Source: CAD feature listing. Evaluate the final solid. Frame: model axes, mm. A direction names the side the tool comes from. Coordinates: 2 decimals unless noted, no trailing zeros. Write each loop counter-clockwise with the first axis right and the second up, starting at its lowest first coordinate (ties: lowest second). Pieces come first, ordered by that corner, then holes. Notation, with made-up numbers: M -10.75,2.5 L 16.25,2.5 A10 ccw 16.25,12.5 Z; hole C -13,74 d9. An arc over 180 degrees is marked long. One line per item, written item: value. Start each with the question number.
Item 1: Cut plane A-A, the plane x = 0. Output: boundary loops of the cut face in (y, z), then the cut area to 3 significant figures.
Item 2: Set-up query: faces 1 (the cylindrical face through (-1.73, -7.81, 107.76)), 2 (the cylindrical face through (-1.64, -7.37, 54.3)). Return all of +Z, -Z, +X, -X, +Y, -Y with unobstructed straight access to the full face (end or side cutting, diameter ignored); none if empty.
Item 3: Pin query (flat end, axial travel): P1, Ø4, axis at x = -4, z = 14.5, coming from the -Y side; P2, Ø4, axis at y = -6.5, z = 60.5, coming from the +X side; P3, Ø2, axis at y = 6.5, z = 64, coming from the +X side. Return the tip coordinate at first contact, or that it passes through.
Item 4: Cut plane C-C, the plane z = 8. Output: boundary loops of the cut face in (x, y).
Item 5: Ray query, L1, parallel to Y at x = 0, z = 107.1; L2, parallel to Y at x = 0.5, z = 53; L3, parallel to X at y = -5.75, z = 26. Return the intervals inside material, ascending. Write a range as from..to.
Item 6: Mould query, pull axis X, two halves, no side actions, for faces 3 (the cylindrical face through (-1.73, -7.81, 2.31)), 4 (the flat face through (-2, 8, 110)), 5 (the cylindrical face through (5.161, 8.095, 54.23)). Classes: released by +X, released by -X, zero draft, split by the parting line, or undercut.
```python
from build123d import *

# Parameters (mm, degrees)
F0_R         = 9.6
F0_R_2       = 8
F1_DEPTH     = 110
F0_R_3       = 7.55
F2_DEPTH     = 106
F3_DEPTH     = 4
F4_S5_R      = 8
F4_T6_DEPTH  = 14
F4_S11_R     = 8
F4_T12_DEPTH = 14


# Not quite as in the source:
# - a fillet or chamfer that OpenCascade refuses, or shapes differently, is made with other operations: its cross-section is extruded or revolved along the edge and cut away or added


with BuildPart() as f1:
    # F0 (on Top) → F1 (new body)
    with BuildSketch(Plane.XY):
        Circle(F0_R)
        Circle(F0_R_2, mode=Mode.SUBTRACT)
    extrude(amount=F1_DEPTH)

    # F0 (on Top) → F2 (join)
    with BuildSketch(Plane.XY):
        Circle(F0_R_2)
        Circle(F0_R_3, mode=Mode.SUBTRACT)
    extrude(amount=F2_DEPTH)

    # F0 (on Top) → F3 (cut)
    with BuildSketch(Plane.XY):
        Circle(F0_R_2)
        Circle(F0_R_3, mode=Mode.SUBTRACT)
    extrude(amount=F3_DEPTH, mode=Mode.SUBTRACT)

    # F4: chamfer of 1 on 2 edges, made by hand


with BuildPart() as f4_tool2:
    # F4_s3 → F4_t4 (revolve)
    with BuildSketch(Plane.XZ):
        Polygon((8.55, 4), (7.55, 5), (7.55, 4), align=None)
    revolve(axis=Axis((0, 0, 4), (0, 0, 1)))

    # F4_s5 → F4_t6 (intersect, symmetric)
    with BuildSketch(Plane.XY.offset(4.5)):
        Circle(F4_S5_R)
    extrude(amount=F4_T6_DEPTH, both=True, mode=Mode.INTERSECT)


with BuildPart() as f1_1:
    add(f1.part)

    # F4_t1: cut F4_tool2
    add(f4_tool2.part, mode=Mode.SUBTRACT)


with BuildPart() as f4_tool8:
    # F4_s9 → F4_t10 (revolve)
    with BuildSketch(Plane.XZ):
        Polygon((8.55, 106), (7.55, 105), (7.55, 106), align=None)
    revolve(axis=Axis((0, 0, 106), (0, 0, 1)))

    # F4_s11 → F4_t12 (intersect, symmetric)
    with BuildSketch(Plane.XY.offset(105.5)):
        Circle(F4_S11_R)
    extrude(amount=F4_T12_DEPTH, both=True, mode=Mode.INTERSECT)


with BuildPart() as f1_2:
    add(f1_1.part)

    # F4_t7: cut F4_tool8
    add(f4_tool8.part, mode=Mode.SUBTRACT)


solid = f1_2.part
```
From the geometry:
1. outline: M -9.6,0 L -8,0 L -8,4.55 L -7.55,5 L -7.55,105 L -8,105.45 L -8,110 L -9.6,110 Z; M 7.55,5 L 8,4.55 L 8,0 L 9.6,0 L 9.6,110 L 8,110 L 8,105.45 L 7.55,105 Z
1. area: 442 mm²
2. face 1: +Z
2. face 2: +Z, -Z
3. P1: stops at y = -9.39
3. P2: stops at x = 8.48
3. P3: stops at x = 7.87
4. outline: C 0,0 d19.2; hole C 0,0 d15.1
5. L1: y = -9.6..-8, 8..9.6
5. L2: y = -9.59..-7.53, 7.53..9.59
5. L3: x = -7.69..-4.89, 4.89..7.69
6. face 3: undercut
6. face 4: zero draft
6. face 5: split by the parting line
